from build123d import *

# Parameters (mm, degrees)
F0_R     = 23
F0_R_2   = 20
F1_DEPTH = 10
F2_R     = 23
F3_DEPTH = 3
F4_R     = 1
F5_R     = 1
F6_R     = 1


with BuildPart() as f1:
    # F0 (on Top) → F1 (new body)
    with BuildSketch(Plane.XY):
        Circle(F0_R)
        Circle(F0_R_2, mode=Mode.SUBTRACT)
    extrude(amount=F1_DEPTH)

    # F2 (on face) → F3 (join)
    with BuildSketch(Plane(origin=(0, 0, 0), x_dir=(1, 0, 0), z_dir=(0, 0, -1))):
        Circle(F2_R)
    extrude(amount=-F3_DEPTH)

    # F4
    f4_edges = [f1.edges().sort_by_distance(p)[0] for p in [
        (-23, 0, 10),
    ]]
    fillet(f4_edges, radius=F4_R)

    # F5
    f5_edges = [f1.edges().sort_by_distance(p)[0] for p in [
        (-20, 0, 10),
    ]]
    fillet(f5_edges, radius=F5_R)

    # F6
    f6_edges = [f1.edges().sort_by_distance(p)[0] for p in [
        (-23, 0, 0),
    ]]
    fillet(f6_edges, radius=F6_R)


solid = f1.part
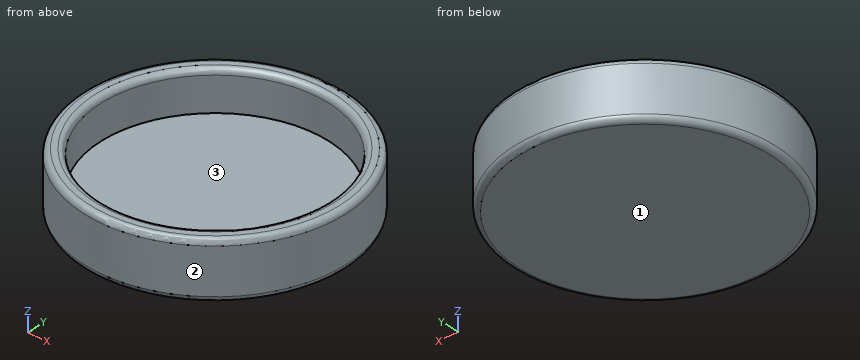
Geometry: final body of the model. Coordinates: model frame, mm. Face numbers are marked on the shaded views. Coordinates: 2 decimals unless noted, no trailing zeros. Loops run counter-clockwise (first coordinate to the right, second up) from the corner with the lowest first, then second, coordinate; pieces in that order, holes last. Notation, with made-up numbers: (-25, -5.5) - (32, -5.5) arc R29 cw to (32, 20.5) - close; hole circle Ø9 at (38.25, 2.5). An arc over 180 degrees is marked (long way). One line per question, with ' | ' between items. Start each with the question number.
(1) Draft query along Z for the marked faces 1, 2 and 3. Return one class per face: +Z half, -Z half, draft (parallel to the pull), parting line (faces both ways), or undercut.
(2) First-contact query: pin 1 (1.5 mm diameter, centred on x = 11, y = -9, fed in from -Z); pin 2 (5 mm diameter, centred on x = -12, y = 6.5, fed in from +Z); pin 3 (6 mm diameter, centred on y = -15, z = 2.5, fed in from -X); pin 4 (5 mm diameter, centred on y = 7.5, z = 7, fed in from +X). Flat tips, straight axial feed; report the tip coordinate or a pass-through.
(3) Cut plane A-A on y = 0. Output: boundary loops of the cut face in (x, z), and give its area (3 significant figures).
(4) Cut plane C-C on z = 6.75. Output: boundary loops of the cut face in (x, y), and give its area (3 significant figures).
(5) Ray query, L1, parallel to Y at x = 0, z = 5.5; L2, parallel to Z at x = -15.5, y = 14; L3, parallel to Z at x = -1.5, y = 11.5. Return the intervals inside material, ascending. Write a range as from..to.
Here are the results:
1) face 1: -Z half | face 2: draft | face 3: +Z half
2) pin 1: z = 0 | pin 2: z = 3 | pin 3: x = -19.62 | pin 4: x = 22.45
3) outline: (-23, 1) arc R1 ccw to (-22, 0) - (22, 0) arc R1 ccw to (23, 1) - (23, 9) arc R1 ccw to (22, 10) - (21, 10) arc R1 ccw to (20, 9) - (20, 3) - (-20, 3) - (-20, 9) arc R1 ccw to (-21, 10) - (-22, 10) arc R1 ccw to (-23, 9) - close | area: 179 mm²
4) outline: circle Ø46 at (0, 0); hole circle Ø40 at (0, 0) | area: 405 mm²
5) L1: -23..-20, 20..23 | L2: 0..9.99 | L3: 0..3
